```python
from build123d import *

# Parameters (mm, degrees)
CYLINDER001_R     = 2
CYLINDER001_DEPTH = 10
CYLINDER_R        = 4
CYLINDER_DEPTH    = 4
FILLET_R          = 1


with BuildPart() as cilindro001:
    # Cylinder001 → Cylinder001 (new body)
    with BuildSketch(Plane(origin=(-35, 16, -2), x_dir=(1, 0, 0), z_dir=(0, 0, 1))):
        Circle(CYLINDER001_R)
    extrude(amount=CYLINDER001_DEPTH)


with BuildPart() as obj1:
    # Cylinder → Cylinder (new body)
    with BuildSketch(Plane(origin=(-35, 16, 0), x_dir=(1, 0, 0), z_dir=(0, 0, 1))):
        Circle(CYLINDER_R)
    extrude(amount=CYLINDER_DEPTH)

    # Cut001: cut Cilindro001
    add(cilindro001.part, mode=Mode.SUBTRACT)


with BuildPart() as obj1_1:
    # Cut001 placement: moved
    add(obj1.part.moved(Location((0, 1.3, 0))))

    # Fillet
    fillet_edges = [obj1_1.edges().sort_by_distance(p)[0] for p in [
        (-39, 17.3, 4),
    ]]
    fillet(fillet_edges, radius=FILLET_R)


with BuildPart() as obj1_2:
    # Fillet placement: moved
    add(obj1_1.part.moved(Location((6, -6, 0))))


solid = obj1_2.part
```
Verification items for the finished model (mm, model axes). Round coordinates to 2 decimals unless told otherwise and drop trailing zeros. Order: outer loops, then holes, each group sorted by start corner. A loop starts at its lowest first (then second) coordinate and runs counter-clockwise, first axis right, second up. Notation, with made-up numbers: (23.25, -15.75) -> (57.25, -15.75) arc R13 ccw to (57.25, 1.25) -> close; hole circle Ø5 at (15.25, 55). An arc over 180 degrees is marked (long way). Put each result on its own line as item: value. Start each with the question number.
(1) Draft check along Y on faces 1 (the face through (-27.153, 10.534, 1.972)), 2 (the face through (-28, 9, 4)), 3 (the face through (-31.95, 14, 1.48)). Enter one of: +Y half, -Y half, draft (parallel to the pull), parting line (faces both ways), or undercut.
(2) Section check A-A (x = -29). Enter the section's corners in (y, z).
(3) Depth check by flat-ended pin: pin 1 Ø3 at (x, y) = (-29, 11.3) entering from +Z; pin 2 Ø1 at (x, y) = (-32, 10) entering from +Z; pin 3 Ø1 at (x, z) = (-26.5, 2.5) entering from +Y; pin 4 Ø1.5 at (y, z) = (10, 2.5) entering from +X. Enter the tip coordinate at first touch or a pass-through.
(4) Material ranges on line 1 along Y through (x, z) = (-29, 2.45); line 2 along Y through (x, z) = (-30.75, 3.3); line 3 along X through (y, z) = (10.25, 3.35), recorded low to high.
(5) Section check B-B (y = 11.3). Enter the section's corners in (x, z), then the cut area to 3 significant figures.
(6) Section check C-C (z = 2.35). Enter the section's corners in (x, y).
Completed:
1. face 1: undercut
1. face 2: draft
1. face 3: parting line
2. outline: (7.3, 0) -> (9.3, 0) -> (9.3, 4) -> (8.3, 4) arc R1 ccw to (7.3, 3) -> close; (13.3, 0) -> (15.3, 0) -> (15.3, 3) arc R1 ccw to (14.3, 4) -> (13.3, 4) -> close
3. pin 1: passes through
3. pin 2: stops at z = 4
3. pin 3: stops at y = 14.76
3. pin 4: stops at x = -25.04
4. line 1: y = 7.3 to 9.3, 13.3 to 15.3
4. line 2: y = 7.75 to 10.33, 12.27 to 14.85
4. line 3: x = -32.79 to -30.7, -27.3 to -25.21
5. outline: (-33, 0) -> (-31, 0) -> (-31, 4) -> (-32, 4) arc R1 ccw to (-33, 3) -> close; (-27, 0) -> (-25, 0) -> (-25, 3) arc R1 ccw to (-26, 4) -> (-27, 4) -> close
5. area: 15.6 mm2
6. outline: circle Ø8 at (-29, 11.3); hole circle Ø4 at (-29, 11.3)
